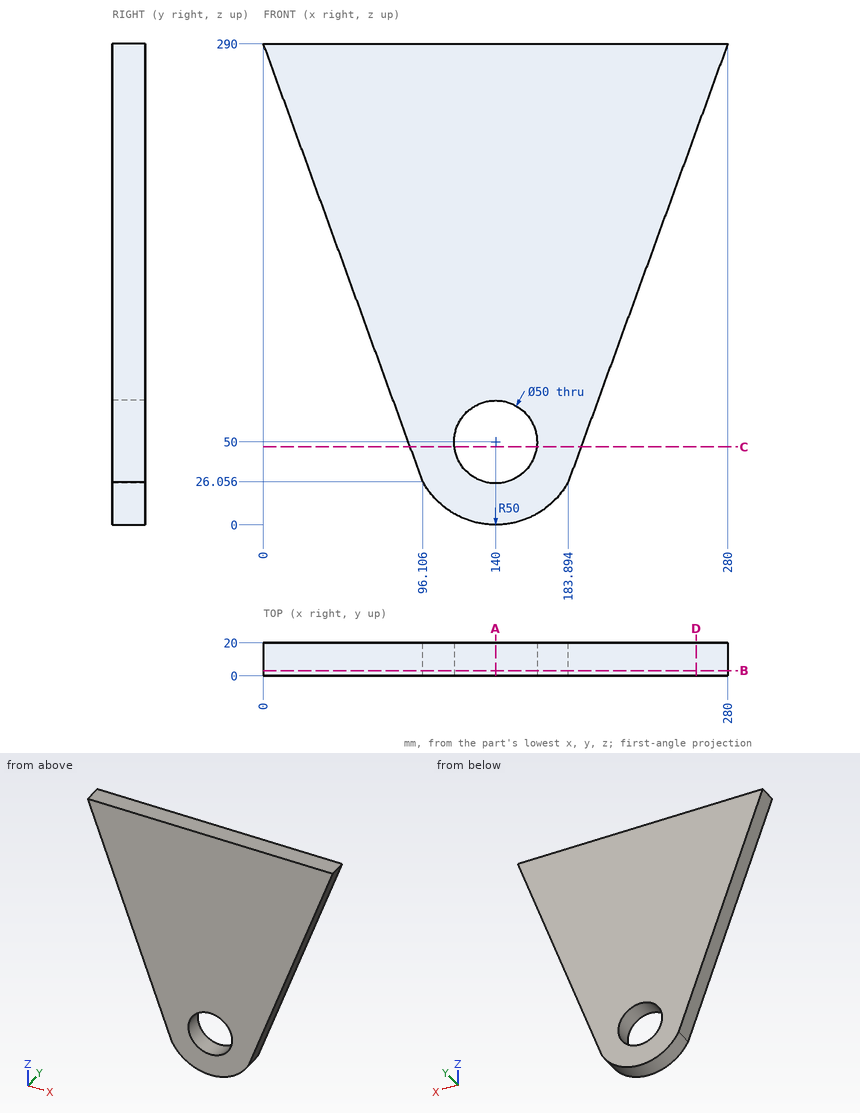
Could you check a few things on this drawing? It's one solid part, dimensions in mm from its lowest x, y, z. Round coordinates to 2 decimals unless told otherwise and drop trailing zeros. Loops run counter-clockwise (first coordinate to the right, second up) from the corner with the lowest first, then second, coordinate; pieces in that order, holes last.
Q1. I want a section at C-C (z = 47). Write out the boundary of the cut face in (x, y).
Q2. I want a section at A-A (x = 140). Write out the boundary of the cut face in (y, z).
Q3. For P1, Ø1, axis at x = 116, y = 17, coming from the -Z side, with a flat end and sliding along its axis, tell me the tip position at first contact or that it passes through.
Q4. I want a section at D-D (x = 261). Write out the boundary of the cut face in (y, z), and give its area (3 significant figures).
Q5. Please list where these lines run through material, in increasing order: L1, parallel to X at y = 9.5, z = 50; L2, parallel to X at y = 8.5, z = 64; L3, parallel to X at y = 5.5, z = 204.
Q6. I want a section at B-B (y = 3.25). Write out the boundary of the cut face in (x, z), and give its area (3 significant figures).
Answer below:
1. outline: (88.48, 0) - (115.18, 0) - (115.18, 20) - (88.48, 20) - close; (164.82, 0) - (191.52, 0) - (191.52, 20) - (164.82, 20) - close
2. outline: (0, 0) - (20, 0) - (20, 25) - (0, 25) - close; (0, 75) - (20, 75) - (20, 290) - (0, 290) - close
3. P1: stops at z = 5.87
4. outline: (0, 237.82) - (20, 237.82) - (20, 290) - (0, 290) - close
4. area: 1,040 mm2
5. L1: x = 87.39 to 115, 165 to 192.61
5. L2: x = 82.29 to 119.29, 160.71 to 197.71
5. L3: x = 31.31 to 248.69
6. outline: (0, 290) - (96.11, 26.06) arc R50 ccw to (183.89, 26.06) - (280, 290) - close; hole circle Ø50 at (140, 50)
6. area: 48,200 mm2
